from build123d import *

# Parameters (mm, degrees)
SKETCH2_R           = 2.55
BOSS_EXTRUDE2_DEPTH = 300
FILLET1_R           = 0.25
FILLET2_R           = 0.25


with BuildPart() as part:
    # Sketch2 → Boss-Extrude2 (new body)
    with BuildSketch(Plane(origin=(0, 0, 0), x_dir=(0, 0, -1), z_dir=(1, 0, 0))):
        Polygon((-20, 13.585786438), (-20, 20), (-13.585786438, 20), (-13.585786438, 18), (-16.585786438, 18), (-12.58578916, 14), (-7.41421084, 14), (-3.414213562, 18), (-6.414213562, 18), (-6.414213562, 20), (0, 20), (0, 18), (-5.414207154, 12.58578916), (-5.414207154, 7.41421084), (0, 2), (0, 0), (-6.414213562, 0), (-6.414213562, 2), (-3.414213562, 2), (-7.41421084, 6), (-12.58578916, 6), (-16.585786438, 2), (-13.585786438, 2), (-13.585786438, 0), (-20, 0), (-20, 6.414213562), (-18, 6.414213562), (-18, 3.414213562), (-14.000005445, 7.41421084), (-14.000005445, 12.58578916), (-18, 16.585786438), (-18, 13.585786438), align=None)
        with Locations((-10, 10)):
            Circle(SKETCH2_R, mode=Mode.SUBTRACT)
    extrude(amount=BOSS_EXTRUDE2_DEPTH)

    # Fillet1
    fillet1_edges = [part.edges().sort_by_distance(p)[0] for p in [
        (150, 13.585786438, 20),
        (150, 20, 20),
        (150, 20, 13.585786438),
        (150, 18, 13.585786438),
        (150, 18, 16.585786438),
        (150, 14, 12.58578916),
        (150, 14, 7.41421084),
        (150, 18, 3.414213562),
        (150, 18, 6.414213562),
        (150, 20, 6.414213562),
        (150, 12.58578916, 5.414207154),
        (150, 7.41421084, 5.414207154),
        (150, 0, 6.414213562),
        (150, 2, 6.414213562),
        (150, 2, 3.414213562),
        (150, 6, 7.41421084),
        (150, 6, 12.58578916),
        (150, 2, 16.585786438),
        (150, 2, 13.585786438),
        (150, 0, 13.585786438),
        (150, 0, 20),
        (150, 6.414213562, 20),
        (150, 6.414213562, 18),
        (150, 3.414213562, 18),
        (150, 7.41421084, 14.000005445),
        (150, 12.58578916, 14.000005445),
        (150, 16.585786438, 18),
        (150, 13.585786438, 18),
    ]]
    fillet(fillet1_edges, radius=FILLET1_R)

    # Mirror3: part across plane


with BuildPart() as part_1:
    add(part.part)
    add(part.part.mirror(Plane(origin=(300, 20, 0), x_dir=(1, 0, 0), z_dir=(0, 0, 1))))

    # Fillet2
    fillet2_edges = [part_1.edges().sort_by_distance(p)[0] for p in [
        (150, 2, 0),
        (150, 18, 0),
    ]]
    fillet(fillet2_edges, radius=FILLET2_R)


solid = part_1.part
For this review, take the finished solid that the model builds, in its own axes (mm). A direction names the side the tool comes from. Coordinates: 2 decimals unless noted, no trailing zeros. Loops run counter-clockwise (first coordinate to the right, second up) from the corner with the lowest first, then second, coordinate; pieces in that order, holes last. Notation, with made-up numbers: (-13.75, 72.5) - (38.25, 72.5) arc R32 ccw to (38.25, 99.5) - close; hole circle Ø7 at (81, -13.75). An arc over 180 degrees is marked (long way). Use a Markdown table: item, result. Add a question column.
Item 1: We need section B-B (z = -10). Give the boundary of the cut face in (x, y), and give its area (3 significant figures).
Item 2: Insertion check: pin 1 Ø2 at (y, z) = (2.5, 11) entering from +X; pin 2 Ø1.5 at (x, z) = (81.5, 9) entering from -Y; pin 3 Ø2.5 at (x, y) = (203, 9.5) entering from +Z; pin 4 Ø5.5 at (x, z) = (104, 11) entering from +Y. Each pin has a flat end and moves straight along its axis. Give the tip position at first contact, or say it passes through.
Item 3: For line 1 (Z direction, x = 252.5, y = 18.75); line 2 (Y direction, x = 122, z = 10); line 3 (Y direction, x = 68, z = -16), list the stretches that pass through material, from the lowest coordinate up.
Item 4: Mouldability with a two-part tool opening along Y and no side actions: class faces 6 (the face through (148, 10, -14)), 7 (the face through (147.9, 7.51, 10.55)), 8 (the face through (148, 14, -10)), 9 (the face through (0, 6, 5)) as pulls with the +Y half, pulls with the -Y half, needs draft (parallel to the pull), parting line crosses it, or undercut.
Item 5: Tool access review of faces 1 (the face through (148, 5, 3)), 2 (the face through (148, 0, 0)), 3 (the face through (148, 20, 17)), 4 (the face through (148, 10, 14)), 5 (the face through (148, 14, 10)): name each direction out of +Z, -Z, +X, -X, +Y, -Y from which nothing blocks a thin tool from reaching the whole face with its end or side.
Item 6: We need section A-A (y = 10). Give the boundary of the cut face in (x, z).
Item 7: We need section C-C (x = 24). Give the number of separate pieces and of enclosed holes in the cut face, and give its area (3 significant figures).
Results list:
| question | item | result |
|---|---|---|
| 1 | outline | (0, 6) - (300, 6) - (300, 7.45) - (0, 7.45) - close; (0, 12.55) - (300, 12.55) - (300, 14) - (0, 14) - close |
| 1 | area | 870 mm^2 |
| 2 | pin 1 | passes through |
| 2 | pin 2 | stops at y = 6 |
| 2 | pin 3 | stops at z = 14 |
| 2 | pin 4 | stops at y = 19.98 |
| 3 | line 1 | z = -20 to -13.59, -6.41 to 6.41, 13.59 to 20 |
| 3 | line 2 | y = 6 to 7.45, 12.55 to 14 |
| 3 | line 3 | y = 0 to 2, 2.59 to 5.41, 14.59 to 17.41, 18 to 20 |
| 4 | face 6 | undercut |
| 4 | face 7 | undercut |
| 4 | face 8 | pulls with the +Y half |
| 4 | face 9 | needs draft |
| 5 | face 1 | +X, -X |
| 5 | face 2 | +Z, -Z, +X, -X, -Y |
| 5 | face 3 | +Z, -Z, +X, -X, +Y |
| 5 | face 4 | +Z, +X, -X |
| 5 | face 5 | +X, -X, +Y |
| 6 | outline | (0, -14) - (300, -14) - (300, -12.55) - (0, -12.55) - close; (0, -7.45) - (300, -7.45) - (300, -5.41) - (0, -5.41) - close; (0, 5.41) - (300, 5.41) - (300, 7.45) - (0, 7.45) - close; (0, 12.55) - (300, 12.55) - (300, 14) - (0, 14) - close |
| 7 | separate pieces | 1 |
| 7 | enclosed holes | 3 |
| 7 | area | 339 mm^2 |
